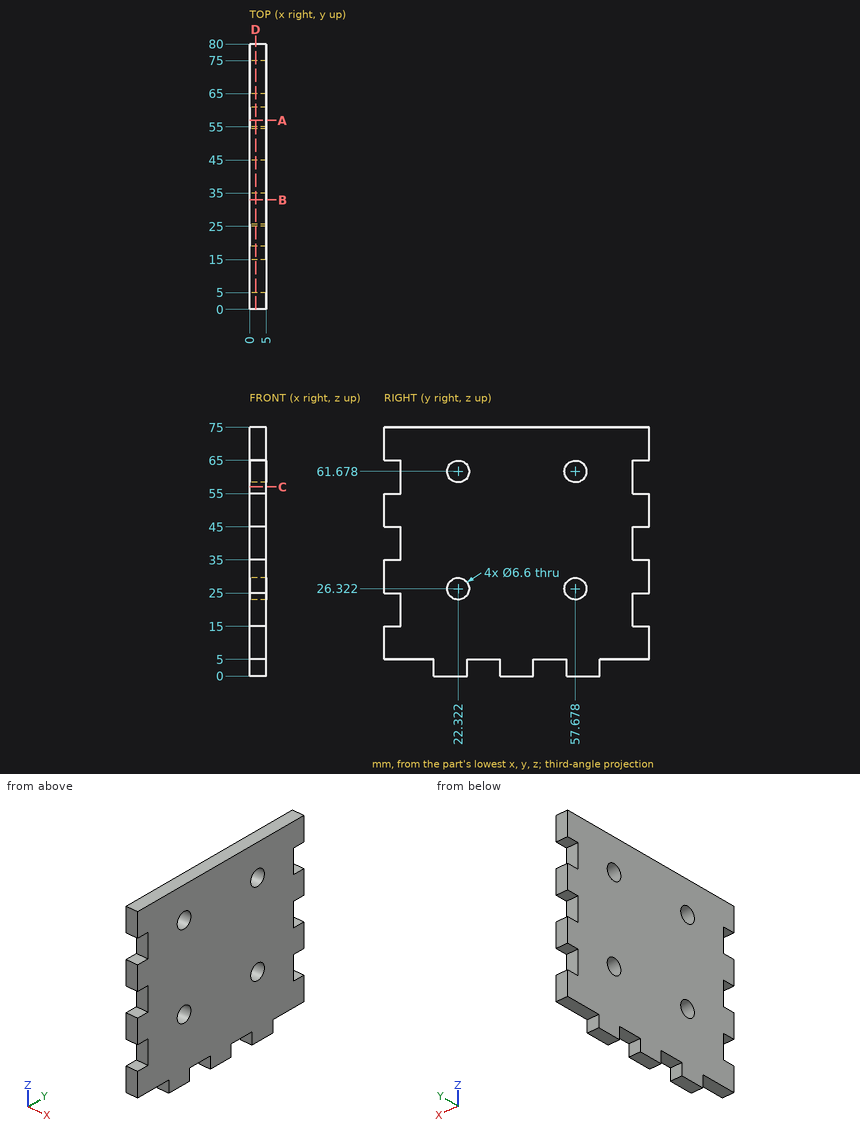
Drawing for the job (mm, zero at the part's lowest x, y, z). Give positions to 0.01 mm unless a question says otherwise; leave off trailing zeros. Order: outer loops, then holes, each group sorted by start corner. A loop starts at its lowest first (then second) coordinate and runs counter-clockwise, first axis right, second up. Notation, with made-up numbers: (18.5, 50.5) -> (59.5, 50.5) arc R18 cw to (59.5, 80.5) -> close; hole circle Ø7 at (-40, -4.5). An arc over 180 degrees is marked (long way). Use one line per item in the form item = value.
(1) Saw through at A-A (y = 57). Write the cut outline in (x, z).
Solution:
outline = (0, 0) -> (5, 0) -> (5, 23.09) -> (0, 23.09) -> close; (0, 29.55) -> (5, 29.55) -> (5, 58.45) -> (0, 58.45) -> close; (0, 64.91) -> (5, 64.91) -> (5, 75) -> (0, 75) -> close
(2) Saw through at B-B (y = 33). Write the cut outline in (x, z), then the cut area to 3 significant figures.
Solution:
outline = (0, 5) -> (5, 5) -> (5, 75) -> (0, 75) -> close
area = 350 mm²
(3) Flat gauge pins, fed straight in: P1, Ø1.5, axis at x = 3.5, z = 3.5, coming from the -Y side; P2, Ø1.5, axis at x = 2, z = 60, coming from the -Y side; P3, Ø2.5, axis at x = 2, z = 3, coming from the +Y side. Where does each tip first touch, or does it go through?
Solution:
P1 = 15
P2 = 5
P3 = 65
(4) Saw through at D-D (x = 1.8). Count the separate pieces of the cut face and the enclosed holes in it, then the cut area to 3 significant figures.
Solution:
separate_pieces = 1
enclosed_holes = 4
area = 5,310 mm²
(5) Drill centre lines: line 1 (Y direction, x = 4.3, z = 4.5); line 2 (Z direction, x = 2.05, y = 20.5) (1 decimal); line 3 (Z direction, x = 1.5, y = 11.5). Where is each one in solid material? Low to high. Write a range as from..to.
Solution:
line_1 = 15..25, 35..45, 55..65
line_2 = 0..23.6, 29.1..58.9, 64.4..75
line_3 = 5..75
